```python
from build123d import *

# Parameters (mm, degrees)
SKETCH1_W           = 109.5
SKETCH1_H           = 50
BOSS_EXTRUDE1_DEPTH = 52.55
SKETCH2_W           = 109.5
SKETCH2_H           = 10
CUT_EXTRUDE1_DEPTH  = 10
SKETCH3_W           = 18.5
SKETCH3_H           = 12
CUT_EXTRUDE2_DEPTH  = 2
FILLET1_R           = 4
SKETCH4_W           = 91
SKETCH4_H           = 5
CUT_EXTRUDE3_DEPTH  = 7
SKETCH5_W           = 23.393715289
SKETCH5_H           = 10
CUT_EXTRUDE4_DEPTH  = 128.873971159
SKETCH6_W           = 94.5
SKETCH6_H           = 10
CUT_EXTRUDE5_DEPTH  = 10
SKETCH8_W           = 18.5
SKETCH8_H           = 12
CUT_EXTRUDE6_DEPTH  = 2
FILLET2_R           = 4
SKETCH9_W           = 76
SKETCH9_H           = 5
CUT_EXTRUDE7_DEPTH  = 7
SKETCH10_R          = 1.5
CUT_EXTRUDE8_DEPTH  = 128.873971159
SKETCH11_R          = 1
CUT_EXTRUDE9_DEPTH  = 7.55
CUT_EXTRUDE10_DEPTH = 132.34592685
FILLET3_R           = 10
SKETCH13_R          = 2.5
CUT_EXTRUDE11_DEPTH = 8
FILLET4_R           = 10
FILLET5_R           = 10
SKETCH15_W          = 63
SKETCH15_H          = 30
SKETCH15_W_2        = 28.5
BOSS_EXTRUDE2_DEPTH = 0.222


with BuildPart() as part:
    # Sketch1 → Boss-Extrude1 (new body)
    with BuildSketch(Plane.XY):
        with Locations((54.75, 25)):
            Rectangle(SKETCH1_W, SKETCH1_H)
    extrude(amount=BOSS_EXTRUDE1_DEPTH)

    # Sketch2 → Cut-Extrude1 (cut)
    with BuildSketch(Plane.XZ):
        with Locations((54.75, 5)):
            Rectangle(SKETCH2_W, SKETCH2_H)
    extrude(amount=-CUT_EXTRUDE1_DEPTH, mode=Mode.SUBTRACT)

    # Sketch3 → Cut-Extrude2 (cut)
    with BuildSketch(Plane.XZ):
        with Locations((9.25, 16)):
            Rectangle(SKETCH3_W, SKETCH3_H)
    extrude(amount=-CUT_EXTRUDE2_DEPTH, mode=Mode.SUBTRACT)

    # Fillet1
    fillet1_edges = [part.edges().sort_by_distance(p)[0] for p in [
        (9.25, 2, 10),
    ]]
    fillet(fillet1_edges, radius=FILLET1_R)

    # Sketch4 → Cut-Extrude3 (cut)
    with BuildSketch(Plane.XZ.offset(-10)):
        with Locations((64, 7.5)):
            Rectangle(SKETCH4_W, SKETCH4_H)
    extrude(amount=-CUT_EXTRUDE3_DEPTH, mode=Mode.SUBTRACT)

    # Sketch5 → Cut-Extrude4 (cut, through all)
    with BuildSketch(Plane.XZ.offset(-10)):
        with Locations((106.196857644, 5)):
            Rectangle(SKETCH5_W, SKETCH5_H)
    extrude(amount=-CUT_EXTRUDE4_DEPTH, mode=Mode.SUBTRACT)

    # Sketch6 → Cut-Extrude5 (cut)
    with BuildSketch(Plane(origin=(0, 50, 0), x_dir=(1, 0, 0), z_dir=(0, 1, 0))):
        with Locations((47.25, -5)):
            Rectangle(SKETCH6_W, SKETCH6_H)
    extrude(amount=-CUT_EXTRUDE5_DEPTH, mode=Mode.SUBTRACT)

    # Sketch8 → Cut-Extrude6 (cut)
    with BuildSketch(Plane(origin=(0, 50, 0), x_dir=(1, 0, 0), z_dir=(0, 1, 0))):
        with Locations((9.25, -16)):
            Rectangle(SKETCH8_W, SKETCH8_H)
    extrude(amount=-CUT_EXTRUDE6_DEPTH, mode=Mode.SUBTRACT)

    # Fillet2
    fillet2_edges = [part.edges().sort_by_distance(p)[0] for p in [
        (9.25, 48, 10),
    ]]
    fillet(fillet2_edges, radius=FILLET2_R)

    # Sketch9 → Cut-Extrude7 (cut)
    with BuildSketch(Plane(origin=(0, 40, 0), x_dir=(1, 0, 0), z_dir=(0, 1, 0))):
        with Locations((56.5, -7.5)):
            Rectangle(SKETCH9_W, SKETCH9_H)
    extrude(amount=-CUT_EXTRUDE7_DEPTH, mode=Mode.SUBTRACT)

    # Sketch10 → Cut-Extrude8 (cut, through all)
    with BuildSketch(Plane(origin=(0, 40, 0), x_dir=(1, 0, 0), z_dir=(0, 1, 0))):
        with Locations((64.5, 0)):
            Circle(SKETCH10_R)
    extrude(amount=-CUT_EXTRUDE8_DEPTH, mode=Mode.SUBTRACT)

    # Sketch11 → Cut-Extrude9 (cut)
    with BuildSketch(Plane.XY.offset(52.55)):
        with Locations((69.5, 15)):
            Circle(SKETCH11_R)
        with Locations((69.5, 35)):
            Circle(SKETCH11_R)
    extrude(amount=-CUT_EXTRUDE9_DEPTH, mode=Mode.SUBTRACT)

    # Sketch12 → Cut-Extrude10 (cut, through all)
    with BuildSketch(Plane(origin=(0, 50, 0), x_dir=(1, 0, 0), z_dir=(0, 1, 0))):
        with BuildLine():
            Line((94.5, -10), (109.5, -10))
            Line((109.5, -10), (109.5, -18.85))
            ThreePointArc((109.5, -18.85), (101.204423403, -15.77343491), (94.5, -10))
        make_face()
    extrude(amount=-CUT_EXTRUDE10_DEPTH, mode=Mode.SUBTRACT)

    # Fillet3
    fillet3_edges = [part.edges().sort_by_distance(p)[0] for p in [
        (109.5, 25, 18.85),
    ]]
    fillet(fillet3_edges, radius=FILLET3_R)

    # Sketch13 → Cut-Extrude11 (cut)
    with BuildSketch(Plane.ZY):
        with Locations((37.552, 35)):
            Circle(SKETCH13_R)
        with Locations((37.552, 15)):
            Circle(SKETCH13_R)
    extrude(amount=-CUT_EXTRUDE11_DEPTH, mode=Mode.SUBTRACT)

    # Fillet4
    fillet4_edges = [part.edges().sort_by_distance(p)[0] for p in [
        (98.648531421, 50, 14.04433448),
        (107.901372758, 50, 20.714757596),
        (109.5, 50, 39.344247885),
    ]]
    fillet(fillet4_edges, radius=FILLET4_R)

    # Fillet5
    fillet5_edges = [part.edges().sort_by_distance(p)[0] for p in [
        (98.648531421, 0, 14.04433448),
        (107.901372758, 0, 20.714757596),
        (109.5, 0, 39.344247885),
    ]]
    fillet(fillet5_edges, radius=FILLET5_R)

    # Sketch15 → Boss-Extrude2 (add)
    with BuildSketch(Plane(origin=(0, 0, 0), x_dir=(-1, 0, 0), z_dir=(0, 0, -1))):
        with Locations((-31.5, 25)):
            Rectangle(SKETCH15_W, SKETCH15_H)
        with Locations((-80.25, 25)):
            Rectangle(SKETCH15_W_2, SKETCH15_H)
    extrude(amount=BOSS_EXTRUDE2_DEPTH)


solid = part.part
```
Source: CAD feature listing. Evaluate the final solid. Frame: model axes, mm. A direction names the side the tool comes from. Coordinates: 2 decimals unless noted, no trailing zeros. Loops run counter-clockwise (first coordinate to the right, second up) from the corner with the lowest first, then second, coordinate; pieces in that order, holes last. Notation, with made-up numbers: M -17.75,22.5 L 24.25,22.5 A20 cw 24.25,52.5 Z; hole C 78,-9 d6. An arc over 180 degrees is marked long. Use CSV: the item, a comma, the result in double quotes.
(1) Contact query for flat-ended pins moving along their axis: pin 1 (6 mm diameter, centred on y = 35, z = 37.552, fed in from -X); pin 2 (2.5 mm diameter, centred on x = 5, z = 18, fed in from +Y); pin 3 (3 mm diameter, centred on y = 29.5, z = 5.5, fed in from +X); pin 4 (9 mm diameter, centred on x = 5, z = 16.5, fed in from -Y). Output: stop coordinate, or through.
Answers follow:
pin 1,"x = 0"
pin 2,"y = 48"
pin 3,"x = 94.5"
pin 4,"y = 2"
(2) Cut plane B-B on z = 39. Return loops of the section in (x, y).
Answers follow:
outline,"M 0,0 L 99.5,0 A10 ccw 109.5,10 L 109.5,40 A10 ccw 99.5,50 L 0,50 L 0,37.04 L 8,37.04 L 8,32.96 L 0,32.96 L 0,17.04 L 8,17.04 L 8,12.96 L 0,12.96 Z"
(3) Cut plane A-A on x = 60.5. Return loops of the section in (y, z), and give its area (3 significant figures).
Answers follow:
outline,"M 0,10 L 17,10 L 17,5 L 10,5 L 10,-0.22 L 40,-0.22 L 40,5 L 33,5 L 33,10 L 50,10 L 50,52.55 L 0,52.55 Z"
area,"2,360 mm²"
(4) Line query: line 1 (Y direction, x = 69.5, z = 50.5); line 2 (Z direction, x = 84, y = 12); line 3 (Z direction, x = 22.5, y = 48). Output: solid intervals per line, ascending. Write a range as [from, to].
Answers follow:
line 1,"[0, 14], [16, 34], [36, 50]"
line 2,"[-0.22, 5], [10, 52.55]"
line 3,"[10, 52.55]"
(5) Reachability of faces 1 (the face through (94.5, 25, 4)), 2 (the face through (18.5, 13, 7)), 3 (the face through (69, 15, 45)), 4 (the face through (9, 49, 22)) from +Z, -Z, +X, -X, +Y, -Y: full face, straight path, thin tool, end or side. Return the list, or none.
Answers follow:
face 1,"-Z, +X, +Y, -Y"
face 2,"+X, -Y"
face 3,"+Z"
face 4,"-Z, -X, +Y"
(6) Draft query along Y for faces 5 (the face through (18.5, 37, 8)), 6 (the face through (3.94, 34.04, 39.86)), 7 (the face through (49, 0, 31)), 8 (the face through (69, 35, 45)). Return one class per face: pulls with the +Y half, pulls with the -Y half, needs draft (parallel to the pull), parting line crosses it, or undercut.
Answers follow:
face 5,"needs draft"
face 6,"undercut"
face 7,"pulls with the -Y half"
face 8,"undercut"
